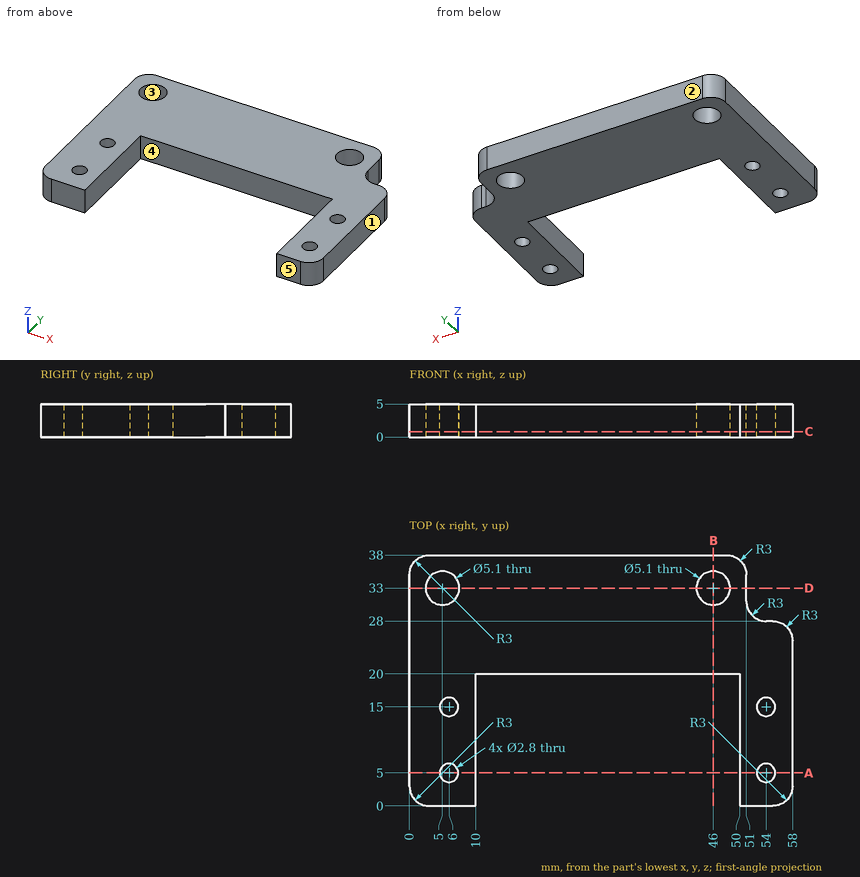
Check sheet for the drawn part. Datum: minimum x, y, z corner. Units: mm. A direction names the side the tool comes from. Round coordinates to 2 decimals unless told otherwise and drop trailing zeros. Order: outer loops, then holes, each group sorted by start corner. A loop starts at its lowest first (then second) coordinate and runs counter-clockwise, first axis right, second up. Notation, with made-up numbers: M 46,7 L 105,7 A24 ccw 105,43 Z; hole C -26.75,19.25 d8. An arc over 180 degrees is marked long. Write each question's results on one line, items separated by ' | '. Start each with the question number.
1. Draft check along Y on the marked faces 1, 2 and 3. Enter one of: pulls with the +Y half, pulls with the -Y half, needs draft (parallel to the pull), parting line crosses it, or undercut.
2. Cross-section at B-B on x = 46. Record the boundary of the cut face in (y, z).
3. Cross-section at D-D on y = 33. Record the boundary of the cut face in (x, z).
4. Cross-section at C-C on z = 0.8. Record the boundary of the cut face in (x, y), plus the area to 3 significant figures.
5. Material ranges on L1, parallel to Y at x = 54, z = 1.15; L2, parallel to X at y = 11, z = 1.1; L3, parallel to X at y = 31.5, z = 3.55, recorded low to high. Write a range as from..to.
6. Set-up check for the marked faces 4 and 5: record each of +Z, -Z, +X, -X, +Y, -Y from which the full face is reachable in a straight line by a thin tool's end or side.
7. Go/stop test with flat-tipped pins: P1, Ø2, axis at y = 27.5, z = 4, coming from the +X side; P2, Ø0.8, axis at x = 54.5, z = 3, coming from the +Y side; P3, Ø1.2, axis at y = 33, z = 2.5, coming from the +X side. Record where each tip stops, or that it passes through.
8. Cross-section at A-A on y = 5. Record the boundary of the cut face in (x, z).
Resolved:
1) face 1: needs draft | face 2: pulls with the +Y half | face 3: undercut
2) outline: M 20,0 L 30.45,0 L 30.45,5 L 20,5 Z; M 35.55,0 L 38,0 L 38,5 L 35.55,5 Z
3) outline: M 0,0 L 2.45,0 L 2.45,5 L 0,5 Z; M 7.55,0 L 43.45,0 L 43.45,5 L 7.55,5 Z; M 48.55,0 L 51,0 L 51,5 L 48.55,5 Z
4) outline: M 0,3 A3 ccw 3,0 L 10,0 L 10,20 L 50,20 L 50,0 L 55,0 A3 ccw 58,3 L 58,25 A3 ccw 55,28 L 54,28 A3 cw 51,31 L 51,35 A3 ccw 48,38 L 3,38 A3 ccw 0,35 Z; hole C 5,33 d5.1; hole C 6,5 d2.8; hole C 6,15 d2.8; hole C 46,33 d5.1; hole C 54,5 d2.8; hole C 54,15 d2.8 | area: 1,260 mm2
5) L1: 0..3.6, 6.4..13.6, 16.4..28 | L2: 0..10, 50..58 | L3: 0..2.94, 7.06..43.94, 48.06..51
6) face 4: +Z, -Z, -Y | face 5: +Z, -Z, +X, -X, -Y
7) P1: x = 57.6 | P2: y = 28 | P3: x = 51
8) outline: M 0,0 L 4.6,0 L 4.6,5 L 0,5 Z; M 7.4,0 L 10,0 L 10,5 L 7.4,5 Z; M 50,0 L 52.6,0 L 52.6,5 L 50,5 Z; M 55.4,0 L 58,0 L 58,5 L 55.4,5 Z
